Autodesk Inventor part; units mm, degrees
ref_plane "YZ Plane" through (0, 0, 0) normal (1, 0, 0) x (0, 1, 0)
ref_plane "XZ Plane" through (0, 0, 0) normal (0, 1, 0) x (-1, 0, 0)
ref_plane "XY Plane" through (0, 0, 0) normal (0, 0, 1) x (1, 0, 0)
sketch "Sketch1" plane through (0, 0, 0) normal (0, 1, 0) x (-1, 0, 0)
  line L0 (-3.175, 0) -> (-3.175, -108.2294)
  line L1 (0, -108.2294) -> (0, 0)
  arc A0 (0, 0) -> (-3.175, 0) centre (-1.5875, 0) ccw
  arc A1 (-3.175, -108.2294) -> (0, -108.2294) centre (-1.5875, -108.2294) ccw
  dimension "d0" = 3.175
  dimension "d1" = 108.2294
extrude "Extrusion1" add sketch "Sketch1" along normal blind 3.81
sketch "Sketch2" plane through (0, 3.81, 0) normal (0, 1, 0) x (1, 0, 0)
  arc A0 (0, 0) -> (3.175, 0) centre (1.5875, 0) ccw
  circle A1 centre (1.5875, 0) radius 0.889
  arc A2 (3.175, 108.2294) -> (0, 108.2294) centre (1.5875, 108.2294) ccw
  circle A3 centre (1.5875, 108.2294) radius 0.889
  dimension "d4" = 1.778
extrude "Extrusion2" cut sketch "Sketch2" against normal blind 3.81
properties part number "scrambler_spider_support2"
Geometry: final body of the model. Coordinates: model frame, mm. Round coordinates to 2 decimals unless told otherwise and drop trailing zeros. Order: outer loops, then holes, each group sorted by start corner. A loop starts at its lowest first (then second) coordinate and runs counter-clockwise, first axis right, second up. Notation, with made-up numbers: M 14.25,68.5 L 41.25,68.5 A25 ccw 41.25,83.5 Z; hole C -27,19.25 d11. An arc over 180 degrees is marked long. One line per item, written item: value.
(1) Cut plane B-B (y = 1.5). Return the cut outline in (x, z) (1 decimal), and give its area (3 significant figures).
Result sheet:
outline: M 0,-108.2 A1.6 ccw 3.2,-108.2 L 3.2,0 A1.6 ccw 0,0 Z; hole C 1.6,-108.2 d1.8; hole C 1.6,0 d1.8
area: 347 mm2
(2) Line query: probe 1 along Z at (x, y) = (1.65, 3); probe 2 along X at (y, z) = (2.3, 0) (1 decimal); probe 3 along Z at (x, y) = (1, 3.65). Output: solid intervals per line, ascending. Write a range as [from, to].
Result sheet:
probe 1: [-109.82, -109.12], [-107.34, -0.89], [0.89, 1.59]
probe 2: [0, 0.7], [2.5, 3.2]
probe 3: [-109.7, -108.9], [-107.56, -0.67], [0.67, 1.47]
(3) Pull-direction query (Z, two-part tool) for faces 1 (the cylindrical face through (1.47, 1.93, -109.11)), 2 (the cylindrical face through (1.553, 1.878, -109.817)), 3 (the flat face through (0, 2, -55)); classes: pulls with the +Z half, pulls with the -Z half, needs draft (parallel to the pull), parting line crosses it, or undercut.
Result sheet:
face 1: undercut
face 2: pulls with the -Z half
face 3: needs draft
(4) Cut plane A-A (x = 1.85). Return the cut outline in (y, z), and give its area (3 significant figures).
Result sheet:
outline: M 0,-109.8 L 3.81,-109.8 L 3.81,-109.08 L 0,-109.08 Z; M 0,-107.38 L 3.81,-107.38 L 3.81,-0.85 L 0,-0.85 Z; M 0,0.85 L 3.81,0.85 L 3.81,1.57 L 0,1.57 Z
area: 411 mm2
(5) Pin query (flat end, axial travel): P1, Ø1, axis at x = 0.5, y = 0.5, coming from the +Z side. Return the tip coordinate at first contact, or that it passes through.
Result sheet:
P1: z = 1.47
